from build123d import *

# Parameters (mm, degrees)
SKETCH_2_R      = 2.25
EXTRUDE_1_DEPTH = 5
FILLET_1_R      = 3


with BuildPart() as part:
    # 草图2 → 凸台-拉伸1 (new body)
    with BuildSketch(Plane(origin=(0, 0, 0), x_dir=(1, 0, 0), z_dir=(0, 1, 0))):
        Polygon((-11.75, 50), (-52.25, 50), (-52.25, 35), (-26.75, 35), (-26.75, 26), (-15, 11), (-15, -50), (15, -50), (15, 11), (26.75, 26), (26.75, 35), (52.25, 35), (52.25, 50), (11.75, 50), (11.75, 26), (-11.75, 26), align=None)
        with Locations(Location((-8, -45.75, 0), (0, 0, 270))):
            Circle(SKETCH_2_R, mode=Mode.SUBTRACT)
        with Locations(Location((0, -45.75, 0), (0, 0, 270))):
            Circle(SKETCH_2_R, mode=Mode.SUBTRACT)
        with Locations(Location((8, -45.75, 0), (0, 0, 270))):
            Circle(SKETCH_2_R, mode=Mode.SUBTRACT)
        with Locations(Location((-8, 21.75, 0), (0, 0, 270))):
            Circle(SKETCH_2_R, mode=Mode.SUBTRACT)
        with Locations(Location((-48, 45.75, 0), (0, 0, 270))):
            Circle(SKETCH_2_R, mode=Mode.SUBTRACT)
        with Locations(Location((-40, 45.75, 0), (0, 0, 270))):
            Circle(SKETCH_2_R, mode=Mode.SUBTRACT)
        with Locations(Location((-32, 45.75, 0), (0, 0, 270))):
            Circle(SKETCH_2_R, mode=Mode.SUBTRACT)
        with Locations(Location((-24, 45.75, 0), (0, 0, 270))):
            Circle(SKETCH_2_R, mode=Mode.SUBTRACT)
        with Locations(Location((-16, 45.75, 0), (0, 0, 270))):
            Circle(SKETCH_2_R, mode=Mode.SUBTRACT)
        with Locations(Location((0, 21.75, 0), (0, 0, 270))):
            Circle(SKETCH_2_R, mode=Mode.SUBTRACT)
        with Locations(Location((8, 21.75, 0), (0, 0, 270))):
            Circle(SKETCH_2_R, mode=Mode.SUBTRACT)
        with Locations(Location((16, 45.75, 0), (0, 0, 270))):
            Circle(SKETCH_2_R, mode=Mode.SUBTRACT)
        with Locations(Location((24, 45.75, 0), (0, 0, 270))):
            Circle(SKETCH_2_R, mode=Mode.SUBTRACT)
        with Locations(Location((32, 45.75, 0), (0, 0, 270))):
            Circle(SKETCH_2_R, mode=Mode.SUBTRACT)
        with Locations(Location((40, 45.75, 0), (0, 0, 270))):
            Circle(SKETCH_2_R, mode=Mode.SUBTRACT)
        with Locations(Location((48, 45.75, 0), (0, 0, 270))):
            Circle(SKETCH_2_R, mode=Mode.SUBTRACT)
    extrude(amount=EXTRUDE_1_DEPTH)

    # 圆角1
    fillet_1_edges = [part.edges().sort_by_distance(p)[0] for p in [
        (15, 2.5, -11),
        (15, 2.5, 50),
        (-15, 2.5, 50),
        (-15, 2.5, -11),
        (-26.75, 2.5, -26),
        (-26.75, 2.5, -35),
        (-52.25, 2.5, -35),
        (-52.25, 2.5, -50),
        (-11.75, 2.5, -50),
        (-11.75, 2.5, -26),
        (11.75, 2.5, -26),
        (11.75, 2.5, -50),
        (52.25, 2.5, -50),
        (52.25, 2.5, -35),
        (26.75, 2.5, -35),
        (26.75, 2.5, -26),
    ]]
    fillet(fillet_1_edges, radius=FILLET_1_R)


solid = part.part
Check sheet for the modelled part. Datum: model origin and axes. Units: mm. A direction names the side the tool comes from. Round coordinates to 2 decimals unless told otherwise and drop trailing zeros. Loops run counter-clockwise (first coordinate to the right, second up) from the corner with the lowest first, then second, coordinate; pieces in that order, holes last. Notation, with made-up numbers: (89.25, 36) - (100.25, 36) arc R11 ccw to (100.25, 53) - close; hole circle Ø3 at (9, -1). An arc over 180 degrees is marked (long way). Answer as CSV lines item,"result". Start each with the question number.
Item 1: Section check C-C (z = -45.75). Count the separate pieces of the cut face and the enclosed holes in it, and give its area (3 significant figures).
Item 2: Section check B-B (z = 45.75). Record the boundary of the cut face in (x, y), and give its area (3 significant figures).
Item 3: Section check A-A (x = -48). Record the boundary of the cut face in (y, z), and give its area (3 significant figures).
Item 4: Release check for a two-part mould opening along Z. For faces 1 (the cylindrical face through (-32, 2, -48)), 2 (the cylindrical face through (-7.901, 2.465, 43.502)), 3 (the flat face through (26.75, 2, -29)), 4 (the cylindrical face through (27.65, 2.54, -34.14)) record: +Z half, -Z half, draft (parallel to the pull), parting line (faces both ways), or undercut.
Item 5: Depth check by flat-ended pin: P1, Ø2.5, axis at y = 3, z = -30, coming from the +X side; P2, Ø3.5, axis at x = 48, z = -45.75, coming from the -Y side; P3, Ø5, axis at x = 32, z = -45.75, coming from the +Y side; P4, Ø1, axis at x = 6.5, y = 1, coming from the -Z side. Enter the tip coordinate at first touch or a pass-through.
Item 6: Set-up check for faces 5 (the flat face through (15, 2, 19)), 6 (the cylindrical face through (10.85, 2.54, -26.86)), 7 (the flat face through (-40, 2, -35)), 8 (the flat face through (0, 2, 50)): record each of +Z, -Z, +X, -X, +Y, -Y from which the full face is reachable in a straight line by a thin tool's end or side.
Item 7: Scan lines: line 1 (X direction, y = 1.4, z = -22); line 2 (X direction, y = 0.35, z = 33.5); line 3 (X direction, y = 0.75, z = -30). Record each from-to range of solid material in increasing order. Write a range as [from, to].
Report:
1,separate pieces,"12"
1,enclosed holes,"0"
1,area,"180 mm2"
2,outline,"(-15, 0) - (-10.25, 0) - (-10.25, 5) - (-15, 5) - close; (-5.75, 0) - (-2.25, 0) - (-2.25, 5) - (-5.75, 5) - close; (2.25, 0) - (5.75, 0) - (5.75, 5) - (2.25, 5) - close; (10.25, 0) - (15, 0) - (15, 5) - (10.25, 5) - close"
2,area,"82.5 mm2"
3,outline,"(0, -50) - (5, -50) - (5, -48) - (0, -48) - close; (0, -43.5) - (5, -43.5) - (5, -35) - (0, -35) - close"
3,area,"52.5 mm2"
4,face 1,"undercut"
4,face 2,"undercut"
4,face 3,"draft"
4,face 4,"+Z half"
5,P1,"stops at x = 26.75"
5,P2,"passes through"
5,P3,"stops at y = 5"
5,P4,"stops at z = -26"
6,face 5,"+Z, +X, +Y, -Y"
6,face 6,"-Z, +Y, -Y"
6,face 7,"+Z, -X, +Y, -Y"
6,face 8,"+Z, +X, -X, +Y, -Y"
7,line 1,"x = [-23.62, -10.24], [-5.76, -2.24], [2.24, 5.76], [10.24, 23.62]"
7,line 2,"x = [-15, 15]"
7,line 3,"x = [-26.75, -11.75], [11.75, 26.75]"
